from build123d import *

# Parameters (mm, degrees)
F1_DEPTH = 50.8
F2_T     = -25.4


with BuildPart() as f1:
    # F0 (on Top) → F1 (new body)
    with BuildSketch(Plane.XY):
        Polygon((87.205826, 322.612249), (-140.567618, 303.190145), (-302.567911, 141.902003), (-322.993317, -85.783664), (-192.286559, -273.330201), (28.393216, -332.982499), (235.78749, -236.828586), (332.854177, -29.859945), (274.174695, 191.080496), align=None)
    extrude(amount=F1_DEPTH)

    # F2
    f2_openings = [f1.faces().sort_by_distance(p)[0] for p in [
        (0, 0, 0),
        (0, 0, 50.8),
    ]]
    offset(amount=F2_T, openings=f2_openings)


solid = f1.part
For this review, take the finished solid that the model builds, in its own axes (mm). A direction names the side the tool comes from. Round coordinates to 2 decimals unless told otherwise and drop trailing zeros. Loops run counter-clockwise (first coordinate to the right, second up) from the corner with the lowest first, then second, coordinate; pieces in that order, holes last. Notation, with made-up numbers: (57, 41) - (84, 41) arc R22 cw to (84, 48) - close; hole circle Ø5 at (-13.75, 88.25). An arc over 180 degrees is marked (long way). Put each result on its own line as item: value. Start each with the question number.
1. Mouldability with a two-part tool opening along Y and no side actions: class faces 1 (the flat face through (-23.057, 287.718, 25.044)), 2 (the flat face through (130.64, -285.58, 25.04)), 3 (the flat face through (-220.43, 223.68, 25.04)) as +Y half, -Y half, draft (parallel to the pull), parting line (faces both ways), or undercut.
2. Insertion check: P1, Ø1.5, axis at x = -128, z = 35.5, coming from the +Y side; P2, Ø5, axis at x = -41.5, z = 8.5, coming from the +Y side; P3, Ø5, axis at x = 12, z = 18, coming from the -Y side. Each pin has a flat end and moves straight along its axis. Give the tip position at first contact, or say it passes through.
3. Consider section C-C on y = 151. State the section outline as (x, z) points.
4. For probe 1 along X at (y, z) = (-243, 33.5); probe 2 along X at (y, z) = (-234, 30); probe 3 along Y at (x, z) = (-100, 30), list the stretches that pass through material, from the lowest coordinate up. Write a range as [from, to].
5. Consider section A-A on x = -111. State the section outline as (y, z) points, plus the area to 3 significant figures.
6. For faces 4 (the flat face through (-287.35, 27.25, 25.04)), 5 (the flat face through (283.641, -134.793, 25.044)), list the 3-axis set-ups (+Z, -Z, +X, -X, +Y, -Y) from which the entire face can be reached by the end or side of a thin tool; tool diameter is ignored.
7. Consider section B-B on z = 8. State the section outline as (x, y) points.
Result sheet:
1. face 1: undercut
1. face 2: -Y half
1. face 3: +Y half
2. P1: y = 304.33
2. P2: y = 311.85
2. P3: y = -329.23
3. outline: (-293.43, 0) - (-257.43, 0) - (-257.43, 50.8) - (-293.43, 50.8) - close; (258.54, 0) - (284.82, 0) - (284.82, 50.8) - (258.54, 50.8) - close
4. probe 1: [-213.42, -182.46], [162.09, 222.48]
4. probe 2: [-219.7, -188.74], [181.5, 237.11]
4. probe 3: [-298.28, -271.96], [281.16, 306.65]
5. outline: (-295.3, 0) - (-268.99, 0) - (-268.99, 50.8) - (-295.3, 50.8) - close; (280.22, 0) - (305.71, 0) - (305.71, 50.8) - (280.22, 50.8) - close
5. area: 2,630 mm^2
6. face 4: +Z, -Z
6. face 5: +Z, -Z, +X, -Y
7. outline: (-322.99, -85.78) - (-192.29, -273.33) - (28.39, -332.98) - (235.79, -236.83) - (332.85, -29.86) - (274.17, 191.08) - (87.21, 322.61) - (-140.57, 303.19) - (-302.57, 141.9) - close; hole (-296.87, -78.85) - (-176.73, -251.22) - (26.1, -306.05) - (216.72, -217.67) - (305.93, -27.44) - (252, 175.63) - (80.15, 296.52) - (-129.2, 278.67) - (-278.1, 130.42) - close
